Read the model definition and answer for the solid it produces. Units are mm, in the model's axes. A direction names the side the tool comes from. Give positions to 0.01 mm unless a question says otherwise; leave off trailing zeros. Write each loop counter-clockwise with the first axis right and the second up, starting at its lowest first coordinate (ties: lowest second). Pieces come first, ordered by that corner, then holes. Notation, with made-up numbers: M 22,46 L 71,46 A10 ccw 71,50 Z; hole C -2,63.25 d2. An arc over 180 degrees is marked long. Write each question's results on one line, items separated by ' | '. Start each with the question number.
```python
from build123d import *

# Parameters (mm, degrees)
SKETCH1_W           = 8
SKETCH1_H           = 2.5
BOSS_EXTRUDE1_DEPTH = 1.75
SKETCH2_W           = 10
SKETCH2_H           = 4.5
BOSS_EXTRUDE2_DEPTH = 0.75
FILLET1_R           = 0.4
FILLET2_R           = 0.4
FILLET3_R           = 1
FILLET4_R           = 0.25


with BuildPart() as part:
    # Sketch1 → Boss-Extrude1 (new body)
    with BuildSketch(Plane(origin=(0, 0, 0), x_dir=(1, 0, 0), z_dir=(0, 1, 0))):
        with Locations((4, 1.25)):
            Rectangle(SKETCH1_W, SKETCH1_H)
    extrude(amount=BOSS_EXTRUDE1_DEPTH)

    # Sketch2 → Boss-Extrude2 (add)
    with BuildSketch(Plane.XZ):
        with Locations((4, -1.25)):
            Rectangle(SKETCH2_W, SKETCH2_H)
    extrude(amount=BOSS_EXTRUDE2_DEPTH)

    # Fillet1
    fillet1_edges = [part.edges().sort_by_distance(p)[0] for p in [
        (0, 0.875, -2.5),
        (0, 0.875, 0),
        (8, 0.875, 0),
        (8, 0.875, -2.5),
    ]]
    fillet(fillet1_edges, radius=FILLET1_R)

    # Fillet2
    fillet2_edges = [part.edges().sort_by_distance(p)[0] for p in [
        (8, 1.75, -1.25),
        (4, 1.75, 0),
        (4, 1.75, -2.5),
        (0, 1.75, -1.25),
        (0.117157288, 1.75, -0.117157288),
        (0.117157288, 1.75, -2.382842712),
        (7.882842712, 1.75, -2.382842712),
        (7.882842712, 1.75, -0.117157288),
    ]]
    fillet(fillet2_edges, radius=FILLET2_R)

    # Fillet3
    fillet3_edges = [part.edges().sort_by_distance(p)[0] for p in [
        (-1, -0.375, 1),
        (-1, -0.375, -3.5),
        (9, -0.375, -3.5),
        (9, -0.375, 1),
    ]]
    fillet(fillet3_edges, radius=FILLET3_R)

    # Fillet4
    fillet4_edges = [part.edges().sort_by_distance(p)[0] for p in [
        (9, 0, -1.25),
        (9, -0.75, -1.25),
        (-1, 0, -1.25),
        (4, 0, 1),
        (4, 0, -3.5),
        (8.707106781, 0, 0.707106781),
        (-0.7071067811865478, 0, 0.7071067811865477),
        (-0.707106781, 0, -3.207106781),
        (8.707106781, 0, -3.207106781),
        (4, -0.75, -3.5),
        (-1, -0.75, -1.25),
        (4, -0.75, 1),
        (8.707106781, -0.75, 0.707106781),
        (-0.707106781, -0.75, 0.707106781),
        (-0.707106781, -0.75, -3.207106781),
        (8.707106781, -0.75, -3.207106781),
    ]]
    fillet(fillet4_edges, radius=FILLET4_R)


solid = part.part
```
Item 1: Section B-B, the plane y = 0.4 is taken. Determine the outline of the cut face in (x, z), then the cut area to 3 significant figures.
Item 2: Section A-A, the plane z = -1.4 is taken. Determine the outline of the cut face in (x, y).
Item 3: Straight lines are drawn through the part: line 1 (Z direction, x = 7.5, y = 0.55); line 2 (X direction, y = 0.6, z = -2.1); line 3 (Y direction, x = 0, z = -2.3). For each, find the intervals that lie inside material, in ascending order.
Item 4: Given P1, Ø1.5, axis at x = 4, y = 1, coming from the -Z side; P2, Ø1.5, axis at x = 3.5, y = 1, coming from the +Z side, each flat-ended and moving along its own axis, determine where each tip first touches the part or whether it passes through.
Item 5: Section C-C, the plane x = 2.5 is taken. Determine the outline of the cut face in (y, z), then the cut area to 3 significant figures.
Item 6: For faces 1 (the flat face through (4, 1, -2.5)), 2 (the flat face through (4, -0.75, -1)), 3 (the flat face through (4, 1, 0)), 4 (the flat face through (8, 1, -1)), 5 (the flat face through (0, 1, -1)), determine the directions among +Z, -Z, +X, -X, +Y, -Y from which every point of the face is accessible in a straight line to the end or side of a thin tool.
Item 7: Section D-D, the plane y = -0.1 is taken. Determine the outline of the cut face in (x, z).
Worked out:
1) outline: M 0,-2.1 A0.4 ccw 0.4,-2.5 L 7.6,-2.5 A0.4 ccw 8,-2.1 L 8,-0.4 A0.4 ccw 7.6,0 L 0.4,0 A0.4 ccw 0,-0.4 Z | area: 19.9 mm²
2) outline: M -1,-0.5 A0.25 ccw -0.75,-0.75 L 8.75,-0.75 A0.25 ccw 9,-0.5 L 9,-0.25 A0.25 ccw 8.75,0 L 8,0 L 8,1.35 A0.4 ccw 7.6,1.75 L 0.4,1.75 A0.4 ccw 0,1.35 L 0,0 L -0.75,0 A0.25 ccw -1,-0.25 Z
3) line 1: z = -2.5 to 0 | line 2: x = 0 to 8 | line 3: y = -0.75 to 0
4) P1: stops at z = -2.5 | P2: stops at z = 0
5) outline: M -0.75,-3.25 A0.25 ccw -0.5,-3.5 L -0.25,-3.5 A0.25 ccw 0,-3.25 L 0,-2.5 L 1.35,-2.5 A0.4 ccw 1.75,-2.1 L 1.75,-0.4 A0.4 ccw 1.35,0 L 0,0 L 0,0.75 A0.25 ccw -0.25,1 L -0.5,1 A0.25 ccw -0.75,0.75 Z | area: 7.63 mm²
6) face 1: -Z, +X, -X, +Y | face 2: +Z, -Z, +X, -X, -Y | face 3: +Z, +X, -X, +Y | face 4: +Z, -Z, +X, +Y | face 5: +Z, -Z, -X, +Y
7) outline: M -0.95,-2.5 A0.95 ccw 0,-3.45 L 8,-3.45 A0.95 ccw 8.95,-2.5 L 8.95,0 A0.95 ccw 8,0.95 L 0,0.95 A0.95 ccw -0.95,0 Z
